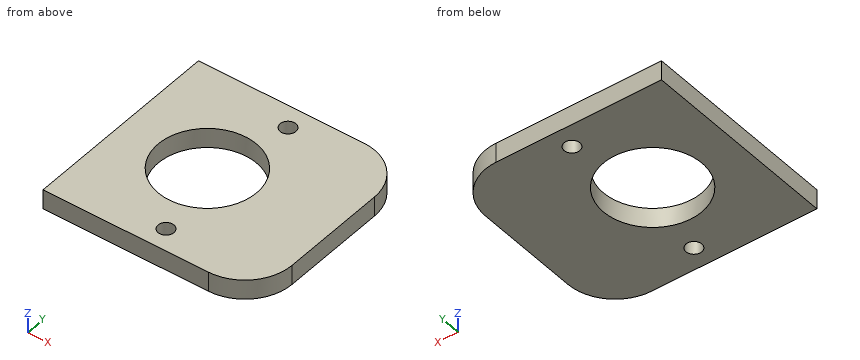
from build123d import *

# Parameters (mm, degrees)
F0_W     = 54
F0_H     = 51
F0_R     = 2
F0_R_2   = 12.5
F1_DEPTH = 5
F2_R     = 12


with BuildPart() as f1:
    # F0 (on Top) → F1 (new body)
    with BuildSketch(Plane.XY):
        Rectangle(F0_W, F0_H)
        with Locations((0, -20)):
            Circle(F0_R, mode=Mode.SUBTRACT)
        with Locations((-5, 0)):
            Circle(F0_R_2, mode=Mode.SUBTRACT)
        with Locations((0, 20)):
            Circle(F0_R, mode=Mode.SUBTRACT)
    extrude(amount=F1_DEPTH)

    # F2
    f2_edges = [f1.edges().sort_by_distance(p)[0] for p in [
        (27, -25.5, 2.5),
        (27, 25.5, 2.5),
    ]]
    fillet(f2_edges, radius=F2_R)


solid = f1.part
Work out the finished part from the listing and answer in its coordinate system (mm). Coordinates: 2 decimals unless noted, no trailing zeros. Write each loop counter-clockwise with the first axis right and the second up, starting at its lowest first coordinate (ties: lowest second). Pieces come first, ordered by that corner, then holes. Notation, with made-up numbers: M 60,-17.75 L 89,-17.75 A20 ccw 89,1.25 Z; hole C 31.5,-16 d5. An arc over 180 degrees is marked long. Answer as CSV lines item,"result". Start each with the question number.
Item 1: Section A-A on x = -12.5 is taken. Write down the section's boundary in (y, z), and give its area (3 significant figures).
Item 2: Section B-B on y = -10 is taken. Write down the section's boundary in (x, z).
Item 3: Consider L1, parallel to Y at x = -5, z = 1.55; L2, parallel to Y at x = 0, z = 3.3; L3, parallel to Y at x = -14.5, z = 2.8. Determine where each line is inside the solid, lowest interval first.
Item 4: Flat-ended cylindrical pins translate along their axes: P1, Ø6, axis at x = -11.5, y = 3.5, coming from the +Z side; P2, Ø1.5, axis at x = 20, z = 2, coming from the +Y side. Find the tip coordinate at first contact, or state that the pin passes through.
Item 5: Section C-C on x = 0 is taken. Write down the section's boundary in (y, z), and give its area (3 significant figures).
Checks:
1,outline,"M -25.5,0 L -10,0 L -10,5 L -25.5,5 Z; M 10,0 L 25.5,0 L 25.5,5 L 10,5 Z"
1,area,"155 mm²"
2,outline,"M -27,0 L -12.5,0 L -12.5,5 L -27,5 Z; M 2.5,0 L 27,0 L 27,5 L 2.5,5 Z"
3,L1,"y = -25.5 to -12.5, 12.5 to 25.5"
3,L2,"y = -25.5 to -22, -18 to -11.46, 11.46 to 18, 22 to 25.5"
3,L3,"y = -25.5 to -8.12, 8.12 to 25.5"
4,P1,"passes through"
4,P2,"stops at y = 24.72"
5,outline,"M -25.5,0 L -22,0 L -22,5 L -25.5,5 Z; M -18,0 L -11.46,0 L -11.46,5 L -18,5 Z; M 11.46,0 L 18,0 L 18,5 L 11.46,5 Z; M 22,0 L 25.5,0 L 25.5,5 L 22,5 Z"
5,area,"100 mm²"
